Autodesk Inventor part; units mm, degrees
ref_plane "YZ Plane" through (0, 0, 0) normal (1, 0, 0) x (0, 1, 0)
ref_plane "XZ Plane" through (0, 0, 0) normal (0, 1, 0) x (-1, 0, 0)
ref_plane "XY Plane" through (0, 0, 0) normal (0, 0, 1) x (1, 0, 0)
sketch "스케치1" plane through (0, 0, 0) normal (0, 0, 1) x (1, 0, 0)
  line L0 (-100, -25) -> (100, -25)
  line L1 (100, -25) -> (100, 25)
  line L2 (100, 25) -> (-100, 25)
  line L3 (-100, 25) -> (-100, -25)
  line L4 (-100, -25) -> (100, 25) construction
  line L5 (100, -25) -> (-100, 25) construction
  line L6 (-25, 22) -> (25, 22)
  line L7 (25, 22) -> (25, 28)
  line L8 (25, 28) -> (-25, 28)
  line L9 (-25, 28) -> (-25, 22)
  line L10 (-25, 22) -> (25, 28) construction
  line L11 (25, 22) -> (-25, 28) construction
  line L12 (-103, -10) -> (-97, -10)
  line L13 (-97, -10) -> (-97, 10)
  line L14 (-97, 10) -> (-103, 10)
  line L15 (-103, 10) -> (-103, -10)
  line L16 (-103, -10) -> (-97, 10) construction
  line L17 (-97, -10) -> (-103, 10) construction
  line L18 (97, -10) -> (103, -10)
  line L19 (103, -10) -> (103, 10)
  line L20 (103, 10) -> (97, 10)
  line L21 (97, 10) -> (97, -10)
  line L22 (97, -10) -> (103, 10) construction
  line L23 (103, -10) -> (97, 10) construction
  point P0 (0, 0)
  point P1 (0, 25)
  point P2 (-100, 0)
  point P3 (100, 0)
  point P4 (-100, -10)
  point P5 (100, -10)
  point P6 (100, 10)
  point P7 (25, 25)
  point P8 (-25, 25)
  point P9 (-100, 10)
  dimension "d0" = 50
  dimension "d1" = 200
  dimension "d2" = 50
  dimension "d3" = 3
  dimension "d4" = 20
  dimension "d5" = 20
  dimension "d6" = 3
  dimension "d7" = 3
extrude "돌출1" add sketch "스케치1" along normal blind 3 contours L3 L12 L13 L14 L2 L9 L6 L7 L1 L20 L21 L18 L0
sketch "스케치2" plane through (0, 0, 3) normal (0, 0, 1) x (1, 0, 0)
  line L0 (-25, -22) -> (25, -22)
  line L1 (25, -22) -> (25, -28)
  line L2 (25, -28) -> (-25, -28)
  line L3 (-25, -28) -> (-25, -22)
  line L4 (-100, -25) -> (100, -25)
  line L5 (-25, -22) -> (25, -28) construction
  line L6 (25, -22) -> (-25, -28) construction
  point P0 (0, 0)
  point P1 (0, -25)
  point P2 (25, -25)
  point P3 (-25, -25)
  dimension "d10" = 50
  dimension "d11" = 3
extrude "돌출2" add sketch "스케치2" against normal blind 3 contours L4 L1 L2 L3
sketch "스케치3" plane through (0, 0, 3) normal (0, 0, 1) x (1, 0, 0)
  point P0 (0, 0)
sketch "스케치4" plane through (0, 0, 3) normal (0, 0, 1) x (1, 0, 0)
  point P0 (0, 0)
sketch "스케치5" plane through (0, 0, 3) normal (0, 0, 1) x (1, 0, 0)
  line L0 (0, 15) -> (-96.3599, 15)
  line L1 (-96.3599, 15) -> (-96.3599, -15)
  line L2 (-96.3599, -15) -> (0, -15)
  line L3 (0, -15) -> (0, 15)
  line L4 (-73.1041, 15) -> (-73.1041, -15)
  line L5 (-25, 25) -> (-100, 25)
  point P0 (0, 0)
  dimension "d14" = 30
  dimension "d15" = 10
extrude "돌출3" cut sketch "스케치5" against normal through all contours L3 L2 L4 L0
properties part number "본체 겉면 레이저 옆판(뚫림) 수정"
Geometry: final body of the model. Coordinates: model frame, mm. Give positions to 0.01 mm unless a question says otherwise; leave off trailing zeros. Write each loop counter-clockwise with the first axis right and the second up, starting at its lowest first coordinate (ties: lowest second). Pieces come first, ordered by that corner, then holes.
(1) Cut plane D-D, the plane x = 65. Return loops of the section in (y, z).
(2) Cut plane B-B, the plane z = 1.95. Return loops of the section in (x, y), then the cut area to 3 significant figures.
(3) Cut plane A-A, the plane y = 8. Return loops of the section in (x, z), then the cut area to 3 significant figures.
(4) Cut plane C-C, the plane x = -45. Return loops of the section in (y, z), then the cut area to 3 significant figures.
(5) First-contact query: P1, Ø1.5, axis at x = -41.5, z = 1, coming from the -Y side; P2, Ø0.9, axis at y = -6, z = 1.5, coming from the -X side; P3, Ø0.9, axis at y = -0.5, z = 1.5, coming from the +X side. Flat tips, straight axial feed; report the tip coordinate or a pass-through.
(6) Ray query, line 1 (Y direction, x = -61, z = 2.15); line 2 (X direction, y = -2.5, z = 1.85); line 3 (Y direction, x = 5, z = 0.85). Return the intervals inside material, ascending.
Values follow:
1. outline: (-25, 0) - (25, 0) - (25, 3) - (-25, 3) - close
2. outline: (-100, -25) - (-25, -25) - (-25, -28) - (25, -28) - (25, -25) - (100, -25) - (100, -10) - (97, -10) - (97, 10) - (100, 10) - (100, 25) - (25, 25) - (25, 22) - (-25, 22) - (-25, 25) - (-100, 25) - (-100, 10) - (-97, 10) - (-97, -10) - (-100, -10) - close; hole (-73.1, -15) - (0, -15) - (0, 15) - (-73.1, 15) - close
2. area: 7,690 mm2
3. outline: (-97, 0) - (-73.1, 0) - (-73.1, 3) - (-97, 3) - close; (0, 0) - (97, 0) - (97, 3) - (0, 3) - close
3. area: 363 mm2
4. outline: (-25, 0) - (-15, 0) - (-15, 3) - (-25, 3) - close; (15, 0) - (25, 0) - (25, 3) - (15, 3) - close
4. area: 60.0 mm2
5. P1: stops at y = -25
5. P2: stops at x = -97
5. P3: stops at x = 97
6. line 1: y = -25 to -15, 15 to 25
6. line 2: x = -97 to -73.1, 0 to 97
6. line 3: y = -28 to 22
